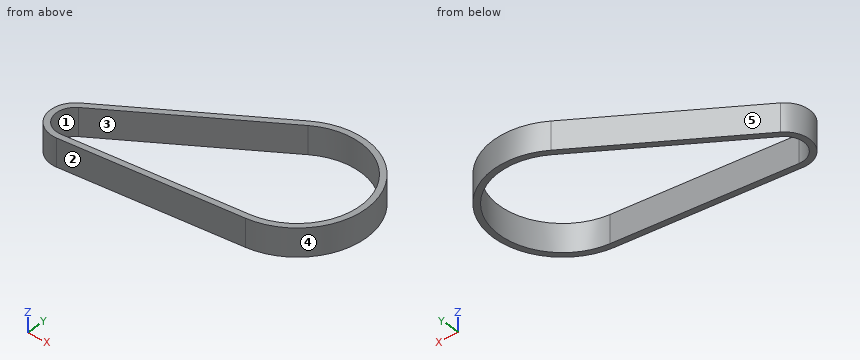
from build123d import *

# Parameters (mm, degrees)
EXTRUS_O_FINA1_DEPTH = 9.53


with BuildPart() as part:
    # Esboço2 → Extrusão-Fina1 (new body)
    with BuildSketch(Plane.XY):
        with BuildLine():
            Line((-63.542787432, -13.379991232), (-12.835941724, 19.684730124))
            ThreePointArc((-12.835941724, 19.684730124), (22.194149255, 7.724619011), (2.159781023, -23.400541573))
            Line((2.159781023, -23.400541573), (-58.118802609, -28.964025676))
            ThreePointArc((-58.118802609, -28.964025676), (-66.927671007, -23.294011131), (-63.542787432, -13.379991232))
        make_face()
        with BuildLine():
            Line((-62.45036686, -15.055287412), (-11.743521152, 18.009433943))
            ThreePointArc((-11.743521152, 18.009433943), (20.305285488, 7.067204627), (1.975969872, -21.40900612))
            Line((1.975969872, -21.40900612), (-58.30261376, -26.972490222))
            ThreePointArc((-58.30261376, -26.972490222), (-65.038807241, -22.636596748), (-62.45036686, -15.055287412))
        make_face(mode=Mode.SUBTRACT)
    extrude(amount=EXTRUS_O_FINA1_DEPTH)


solid = part.part
For this review, take the finished solid that the model builds, in its own axes (mm). Face numbers are marked on the shaded views. A direction names the side the tool comes from. Round coordinates to 2 decimals unless told otherwise and drop trailing zeros. Loops run counter-clockwise (first coordinate to the right, second up) from the corner with the lowest first, then second, coordinate; pieces in that order, holes last. Notation, with made-up numbers: (-38, -18) - (9, -18) arc R31 ccw to (9, 14) - close; hole circle Ø9 at (70, 3.25). An arc over 180 degrees is marked (long way). One line per item, written item: value. Start each with the question number.
Item 1: Take a section at C-C (x = 1). Give the boundary of the cut face in (y, z), plus the area to 3 significant figures.
Item 2: Clearance check with flat-ended pins moving along their axes: pin 1 Ø1 at (y, z) = (-7, 2) entering from -X; pin 2 Ø8 at (x, y) = (-23, 7) entering from +Z; pin 3 Ø5 at (y, z) = (-3.5, 5) entering from +X; pin 4 Ø2 at (x, z) = (-43, 7.5) entering from +Y. State where each tip first meets the part, or that it passes through.
Item 3: For L1, parallel to Y at x = 0, z = 7.25; L2, parallel to X at y = 0, z = 6.5; L3, parallel to X at y = 0.5, z = 4.5, list the stretches that pass through material, from the lowest coordinate up.
Item 4: Take a section at A-A (z = 5). Give the boundary of the cut face in (x, y), plus the area to 3 significant figures.
Item 5: The part is to be moulded in two halves that separate along X. For the marked faces 3, 4 and 5, say which applies: +X half, -X half, draft (parallel to the pull), parting line (faces both ways), or undercut.
Item 6: For the marked faces 1 and 2, list the 3-axis set-ups (+Z, -Z, +X, -X, +Y, -Y) from which the entire face can be reached by the end or side of a thin tool; tool diameter is ignored.
Item 7: Take a section at B-B (y = -20). Give the boundary of the cut face in (x, z), plus the area to 3 significant figures.
Answer below:
1. outline: (-23.51, 0) - (-21.5, 0) - (-21.5, 9.53) - (-23.51, 9.53) - close; (21.48, 0) - (23.48, 0) - (23.48, 9.53) - (21.48, 9.53) - close
1. area: 38.2 mm2
2. pin 1: stops at x = -54.53
2. pin 2: stops at z = 9.53
2. pin 3: stops at x = 23.48
2. pin 4: stops at y = 0.67
3. L1: y = -23.6 to -21.59, 21.5 to 23.5
3. L2: x = -43.02 to -39.36, 21.5 to 23.5
3. L3: x = -42.26 to -38.6, 21.49 to 23.49
4. outline: (-63.54, -13.38) arc R8.5 ccw to (-58.12, -28.96) - (2.16, -23.4) arc R23.5 ccw (long way) to (-12.84, 19.68) - close; hole (-62.45, -15.06) arc R6.5 ccw to (-58.3, -26.97) - (1.98, -21.41) arc R21.5 ccw (long way) to (-11.74, 18.01) - close
4. area: 445 mm2
5. face 3: undercut
5. face 4: parting line
5. face 5: -X half
6. face 1: +Z, -Z
6. face 2: +Z, -Z, +X, -Y
7. outline: (-67.39, 0) - (-65.38, 0) - (-65.38, 9.53) - (-67.39, 9.53) - close; (7.89, 0) - (12.34, 0) - (12.34, 9.53) - (7.89, 9.53) - close
7. area: 61.5 mm2
